Geometry: see drawing. Coordinates: mm, zero at the bounding-box minimum. Coordinates: 2 decimals unless noted, no trailing zeros. Order: outer loops, then holes, each group sorted by start corner. A loop starts at its lowest first (then second) coordinate and runs counter-clockwise, first axis right, second up. Notation, with made-up numbers: (-3, 22) -> (33, 22) arc R20 ccw to (33, 33) -> close; hole circle Ø2 at (87.5, 69.25). An arc over 180 degrees is marked (long way). Use CSV: the item, a comma, the result in double quotes. Start each with the question number.
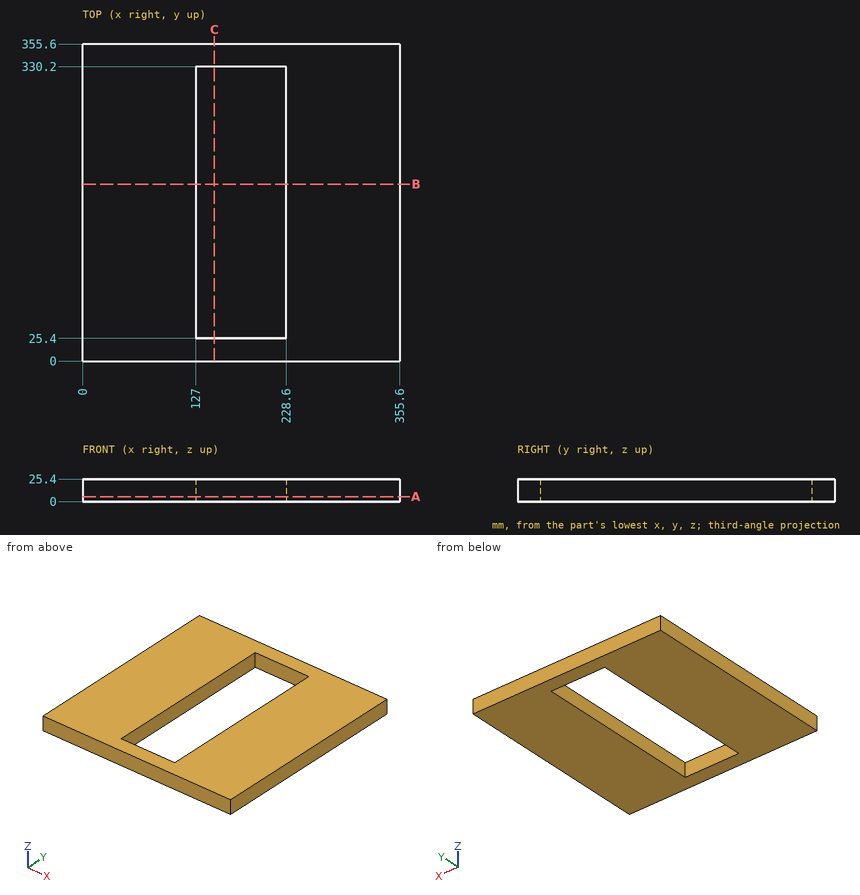
(1) Section A-A (z = 5.5). Return loops of the section in (x, y), then the cut area to 3 significant figures.
(2) Section C-C (x = 148). Return loops of the section in (y, z).
(3) Line query: line 1 (X direction, y = 112, z = 17.75); line 2 (Y direction, x = 217, z = 7.5). Output: solid intervals per line, ascending. Write a range as from..to.
(4) Section B-B (y = 198.5). Return loops of the section in (x, z), then the cut area to 3 significant figures.
Check sheet entries:
1,outline,"(0, 0) -> (355.6, 0) -> (355.6, 355.6) -> (0, 355.6) -> close; hole (127, 25.4) -> (228.6, 25.4) -> (228.6, 330.2) -> (127, 330.2) -> close"
1,area,"95,500 mm^2"
2,outline,"(0, 0) -> (25.4, 0) -> (25.4, 25.4) -> (0, 25.4) -> close; (330.2, 0) -> (355.6, 0) -> (355.6, 25.4) -> (330.2, 25.4) -> close"
3,line 1,"x = 0..127, 228.6..355.6"
3,line 2,"y = 0..25.4, 330.2..355.6"
4,outline,"(0, 0) -> (127, 0) -> (127, 25.4) -> (0, 25.4) -> close; (228.6, 0) -> (355.6, 0) -> (355.6, 25.4) -> (228.6, 25.4) -> close"
4,area,"6,450 mm^2"
